Verification items for this drawing (mm, ordinates from the low corner). A direction names the side the tool comes from. Coordinates: 2 decimals unless noted, no trailing zeros. Order: outer loops, then holes, each group sorted by start corner. A loop starts at its lowest first (then second) coordinate and runs counter-clockwise, first axis right, second up. Notation, with made-up numbers: M 44,-14 L 88,-14 A16 cw 88,16 Z; hole C 7.5,9 d11. An arc over 180 degrees is marked long. Answer as a JSON object with one key per item and string values. Group by question number.
(1) Cross-section at A-A (y = 45). Enter the section's corners in (x, z).
(2) Cross-section at C-C (z = 5.25). Enter the section's corners in (x, y).
(3) Material ranges on line 1 (Y direction, x = 49.25, z = 1.65); line 2 (X direction, y = 37, z = 8.25); line 3 (Y direction, x = 4, z = 2.25), recorded low to high.
(4) Cross-section at D-D (y = 26.5). Enter the section's corners in (x, z).
(5) Cross-section at B-B (x = 37.5). Enter the section's corners in (y, z).
(6) Mould release check, pull along X, two halves, no side actions. Record for the marked faces 1, 2 and 3: released by +X, released by -X, zero draft, split by the parting line, or undercut.
(7) Access from +Z, -Z, +X, -X, +Y, -Y to the whole of each face (thin tool, end or side, straight path). Record for the marked faces 4 and 5.
(8) Gauge pin test, flat ends, axial feed: pin 1 Ø10 at (x, z) = (32.5, 19.5) entering from -Y; pin 2 Ø5 at (x, z) = (15.5, 19) entering from +Y; pin 3 Ø12 at (x, y) = (62.5, 10) entering from +Z. Record the tip position at first contact, or that the pin passes through.
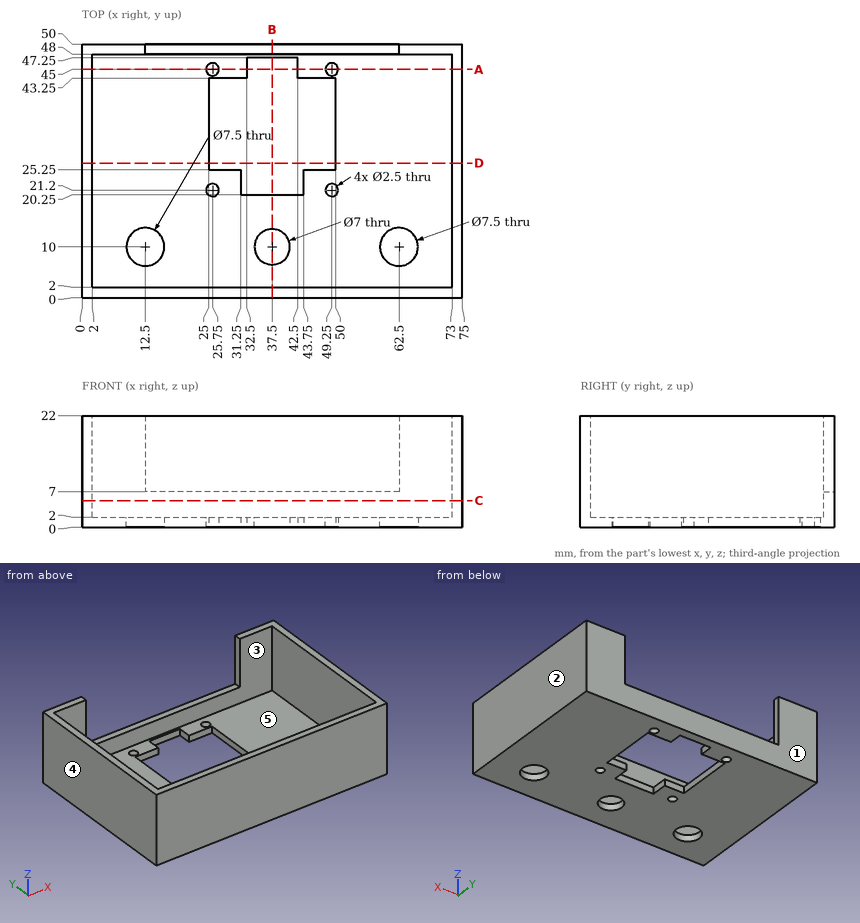
Taken from the geometry:
{
 "1": {"outline": "M 0,0 L 24.5,0 L 24.5,2 L 2,2 L 2,22 L 0,22 Z; M 27,0 L 32.5,0 L 32.5,2 L 27,2 Z; M 42.5,0 L 48,0 L 48,2 L 42.5,2 Z; M 50.5,0 L 75,0 L 75,22 L 73,22 L 73,2 L 50.5,2 Z"},
 "2": {"outline": "M 0,0 L 75,0 L 75,50 L 0,50 Z; hole M 2,2 L 73,2 L 73,48 L 2,48 Z"},
 "3": {"line 1": "y = 0 to 19.95, 22.45 to 25.25, 43.25 to 43.75, 46.25 to 50", "line 2": "x = 0 to 2, 73 to 75", "line 3": "y = 0 to 2, 48 to 50"},
 "4": {"outline": "M 0,0 L 25,0 L 25,2 L 2,2 L 2,22 L 0,22 Z; M 50,0 L 75,0 L 75,22 L 73,22 L 73,2 L 50,2 Z"},
 "5": {"outline": "M 0,0 L 6.5,0 L 6.5,2 L 2,2 L 2,22 L 0,22 Z; M 13.5,0 L 20.25,0 L 20.25,2 L 13.5,2 Z; M 47.25,0 L 50,0 L 50,7 L 48,7 L 48,2 L 47.25,2 Z"},
 "6": {"face 1": "zero draft", "face 2": "released by +X", "face 3": "undercut"},
 "7": {"face 4": "+Z, -Z, -X, +Y, -Y", "face 5": "+Z"},
 "8": {"pin 1": "stops at y = 0", "pin 2": "stops at y = 2", "pin 3": "stops at z = 2"}
}
